For this review, take the finished solid that the model builds, in its own axes (mm). Face numbers are marked on the shaded views. A direction names the side the tool comes from. Coordinates: 2 decimals unless noted, no trailing zeros. Write each loop counter-clockwise with the first axis right and the second up, starting at its lowest first coordinate (ties: lowest second). Pieces come first, ordered by that corner, then holes. Notation, with made-up numbers: (-25, -31) - (20, -31) arc R26 ccw to (20, -8) - close; hole circle Ø1 at (-38, 75.5). An arc over 180 degrees is marked (long way). Use one line per item in the form item = value. Start each with the question number.
1) For L1, parallel to X at y = -48, z = 15.5; L2, parallel to Y at x = 15, z = 36; L3, parallel to Y at x = 27, z = 13, list the stretches that pass through material, from the lowest coordinate up. Write a range as from..to.
2) Mouldability with a two-part tool opening along X and no side actions: class the marked faces 4, 5 and 6 as pulls with the +X half, pulls with the -X half, needs draft (parallel to the pull), parting line crosses it, or undercut.
3) We need section A-A (y = -51). Give the boundary of the cut face in (x, z).
4) We need section B-B (x = 8.5). Give the boundary of the cut face in (y, z).
5) We need section C-C (y = -7). Give the boundary of the cut face in (x, z).
6) We need section D-D (z = 18). Give the boundary of the cut face in (x, y), plus the area to 3 significant figures.
7) Insertion check: P1, Ø10, axis at x = 52.5, z = 7, coming from the -Y side; P2, Ø14, axis at x = 51, z = 37, coming from the -Y side. Each pin has a flat end and moves straight along its axis. Give the tip position at first contact, or say it passes through.
8) Tool access review of the marked faces 1, 2 and 3: name each direction out of +Z, -Z, +X, -X, +Y, -Y from which nothing blocks a thin tool from reaching the whole face with its end or side.
```python
from build123d import *

# Parameters (mm, degrees)
F1_DEPTH = 95
F3_DEPTH = 10
F4_W     = 57
F4_H     = 24
F5_DEPTH = 55.8


with BuildPart() as f1:
    # F0 (on Right) → F1 (new body)
    with BuildSketch(Plane.YZ):
        Polygon((0, 56), (-10, 56), (-10, 28), (-60.793455, 13), (-60.793455, 0), (-10, 0), (0, 0), (0, 28), align=None)
    extrude(amount=F1_DEPTH)

    # F2 (on face) → F3 (cut, through all)
    with BuildSketch(Plane.XZ.offset(10)):
        Polygon((95, 56), (57, 56), (95, 28), align=None)
    extrude(amount=-F3_DEPTH, mode=Mode.SUBTRACT)

    # F4 (on face) → F5 (cut)
    with BuildSketch(Plane(origin=(0, 0, 0), x_dir=(1, 0, 0), z_dir=(0, 0, -1))):
        with Locations((47.5, 48.793455)):
            Rectangle(F4_W, F4_H)
    extrude(amount=-F5_DEPTH, mode=Mode.SUBTRACT)


solid = f1.part
```
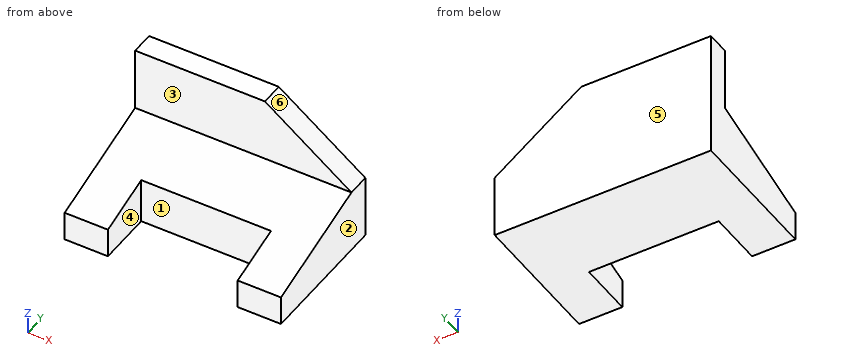
Determined:
q1.L1 = 0..19, 76..95
q1.L2 = -10..0
q1.L3 = -36.79..0
q2.face_4 = undercut
q2.face_5 = needs draft
q2.face_6 = pulls with the +X half
q3.outline = (0, 0) - (19, 0) - (19, 15.89) - (0, 15.89) - close; (76, 0) - (95, 0) - (95, 15.89) - (76, 15.89) - close
q4.outline = (-60.79, 0) - (0, 0) - (0, 56) - (-10, 56) - (-10, 28) - (-60.79, 13) - close
q5.outline = (0, 0) - (95, 0) - (95, 28) - (57, 56) - (0, 56) - close
q6.outline = (0, -43.86) - (19, -43.86) - (19, -36.79) - (76, -36.79) - (76, -43.86) - (95, -43.86) - (95, 0) - (0, 0) - close
q6.area = 3,760 mm²
q7.P1 = -36.79
q7.P2 = -10
q8.face_1 = +Z, -Z, -Y
q8.face_2 = +Z, -Z, +X, +Y, -Y
q8.face_3 = +Z, +X, -X, -Y
